from build123d import *

# Parameters (mm, degrees)
SKETCH013_R      = 4.103857
EXTRUDE012_DEPTH = 120
SKETCH012_R      = 4.612338
EXTRUDE011_DEPTH = 90
SKETCH031_W      = 3.449714
SKETCH031_H      = 1.767909
EXTRUDE033_DEPTH = 70
SKETCH174_R      = 1.623797
EXTRUDE193_DEPTH = 10
SKETCH176_R      = 2.9
EXTRUDE005_DEPTH = 50
EXTRUDE002_DEPTH = 2


with BuildPart() as extrude012:
    # Sketch013 → Extrude012 (new body)
    with BuildSketch(Plane.XZ):
        with Locations((70, 3.549289)):
            Circle(SKETCH013_R)
    extrude(amount=EXTRUDE012_DEPTH)


with BuildPart() as extrude012_1:
    # Extrude012 placement: moved
    add(extrude012.part.moved(Location((0, 105, 0))))


with BuildPart() as tubo:
    # Sketch012 → Extrude011 (new body)
    with BuildSketch(Plane.XZ):
        with Locations((70, 3.62)):
            Circle(SKETCH012_R)
    extrude(amount=EXTRUDE011_DEPTH)


with BuildPart() as tubo_1:
    # Extrude011 placement: moved
    add(tubo.part.moved(Location((0, 90, 0))))

    # Cut004: cut Extrude012
    add(extrude012_1.part, mode=Mode.SUBTRACT)


with BuildPart() as fusion066:
    # Sketch031 → Extrude033 (new body)
    with BuildSketch(Plane.XZ):
        with Locations((69.96706, -1.473137)):
            Rectangle(SKETCH031_W, SKETCH031_H)
    extrude(amount=EXTRUDE033_DEPTH)


with BuildPart() as fusion066_1:
    # Extrude033 placement: moved
    add(fusion066.part.moved(Location((0, 80, 0))))

    # Fusion066: union Tubo
    add(tubo_1.part)


with BuildPart() as fusion066_2:
    # Fusion066 placement: moved
    add(fusion066_1.part.moved(Location((0, 0, -8.2))))


with BuildPart() as extrude193:
    # Sketch174 (on Face4 of Cut014) → Extrude193 (new body)
    with BuildSketch(Plane.XY.offset(12.1)):
        with Locations((30, 86.963425)):
            Circle(SKETCH174_R)
        with Locations((30, 3.252438)):
            Circle(SKETCH174_R)
        with Locations((95.163345, 10)):
            Circle(SKETCH174_R)
        with Locations((94.949776, 80)):
            Circle(SKETCH174_R)
        with Locations((117.10096, 20)):
            Circle(SKETCH174_R)
        with Locations((117.030609, 70)):
            Circle(SKETCH174_R)
        with Locations((117.10096, 44.443623)):
            Circle(SKETCH174_R)
    extrude(amount=EXTRUDE193_DEPTH)


with BuildPart() as extrude193_1:
    # Extrude193 placement: moved
    add(extrude193.part.moved(Location((0, 0, -27.7))))


with BuildPart() as tornillos002:
    # Sketch176 (on Face8 of Extrude002) → Extrude005 (new body)
    with BuildSketch(Plane.XY.offset(2)):
        with Locations((10, 80.016689)):
            Circle(SKETCH176_R)
        with Locations((10, 45.008344)):
            Circle(SKETCH176_R)
        with Locations((10, 10)):
            Circle(SKETCH176_R)
    extrude(amount=EXTRUDE005_DEPTH)


with BuildPart() as tornillos002_1:
    # Extrude005 placement: moved
    add(tornillos002.part.moved(Location((0, 0, -21))))


with BuildPart() as base:
    # Sketch175 → Extrude002 (new body)
    with BuildSketch(Plane.XY):
        Polygon((0, 0), (30, 0), (120, 10), (120, 80), (30, 90), (0, 90), align=None)
    extrude(amount=EXTRUDE002_DEPTH)

    # Cut002: cut Tornillos002
    add(tornillos002_1.part, mode=Mode.SUBTRACT)


with BuildPart() as base_1:
    # Cut002 placement: moved
    add(base.part.moved(Location((0, 0, -12))))

    # Cut122: cut Extrude193
    add(extrude193_1.part, mode=Mode.SUBTRACT)

    # Fusion065: union Fusion066
    add(fusion066_2.part)


with BuildPart() as base_2:
    # Fusion065 placement: moved
    add(base_1.part.moved(Location((0, 0, 15.3))))


solid = base_2.part
The model under review builds one solid part; all positions refer to its coordinate system, in mm. Give positions to 0.01 mm unless a question says otherwise; leave off trailing zeros. Loops run counter-clockwise (first coordinate to the right, second up) from the corner with the lowest first, then second, coordinate; pieces in that order, holes last. Notation, with made-up numbers: (86, -3) -> (115, -3) arc R13 ccw to (115, 16) -> close; hole circle Ø10 at (29.5, 43.5). An arc over 180 degrees is marked (long way). Answer as a JSON object with one key per item and string values. Group by question number.
Q1. Insertion check: pin 1 (3 mm diameter, centred on x = 30, y = 3.25, fed in from +Z); pin 2 (4 mm diameter, centred on y = 30.5, z = 13.5, fed in from +X); pin 3 (1.2 mm diameter, centred on y = 38.5, z = 5.5, fed in from +X); pin 4 (6.5 mm diameter, centred on x = 10, y = 10, fed in from +Z). Each pin has a flat end and moves straight along its axis. Give the tip position at first contact, or say it passes through.
Q2. Take a section at D-D (x = 43). Write out the cut boundary in (y, z).
Q3. Wall thickness on line 1 along Y through (x, z) = (10, 4.2); line 2 along Z through (x, y) = (73, 22); line 3 along X through (y, z) = (50, 11): over which ranges is each line inside the solid? List them lowest first.
Q4. Draft analysis for pull direction X (two halves, no side actions). For faces 1 (the flat face through (59, 46, 3.3)), 2 (the cylindrical face through (118.53, 69.38, 4.29)), 3 (the flat face through (74.37, 4.93, 4.29)), state which applies: pulls with the +X half, pulls with the -X half, needs draft (parallel to the pull), parting line crosses it, or undercut.
Q5. Take a section at B-B (y = 15.5). Write out the cut boundary in (x, z), plus the area to 3 significant figures.
Q6. Take a section at A-A (x = 10). Write out the cut boundary in (y, z).
Q7. Take a section at C-C (x = 70). Write out the cut boundary in (y, z), plus the area to 3 significant figures.
Answer below:
{
 "1": {"pin 1": "passes through", "pin 2": "stops at x = 74.55", "pin 3": "stops at x = 120", "pin 4": "stops at z = 5.3"},
 "2": {"outline": "(1.44, 3.3) -> (88.56, 3.3) -> (88.56, 5.3) -> (1.44, 5.3) -> close"},
 "3": {"line 1": "y = 0 to 7.1, 12.9 to 42.11, 47.91 to 77.12, 82.92 to 90", "line 2": "z = 3.3 to 5.3, 7.22 to 7.85, 13.45 to 14.22", "line 3": "x = 65.4 to 65.91, 74.09 to 74.6"},
 "4": {"face 1": "needs draft", "face 2": "undercut", "face 3": "pulls with the +X half"},
 "5": {"outline": "(0, 3.3) -> (120, 3.3) -> (120, 5.3) -> (71.69, 5.3) -> (71.69, 6.43) arc R4.61 ccw (long way) to (68.24, 6.46) -> (68.24, 5.3) -> (0, 5.3) -> close; hole circle Ø8.21 at (70, 10.65)", "area": "257 mm2"},
 "6": {"outline": "(0, 3.3) -> (7.1, 3.3) -> (7.1, 5.3) -> (0, 5.3) -> close; (12.9, 3.3) -> (42.11, 3.3) -> (42.11, 5.3) -> (12.9, 5.3) -> close; (47.91, 3.3) -> (77.12, 3.3) -> (77.12, 5.3) -> (47.91, 5.3) -> close; (82.92, 3.3) -> (90, 3.3) -> (90, 5.3) -> (82.92, 5.3) -> close"},
 "7": {"outline": "(0, 6.11) -> (10, 6.11) -> (10, 5.3) -> (4.44, 5.3) -> (4.44, 3.3) -> (85.56, 3.3) -> (85.56, 5.3) -> (80, 5.3) -> (80, 6.11) -> (90, 6.11) -> (90, 6.55) -> (0, 6.55) -> close; (0, 14.75) -> (90, 14.75) -> (90, 15.33) -> (0, 15.33) -> close", "area": "310 mm2"}
}
